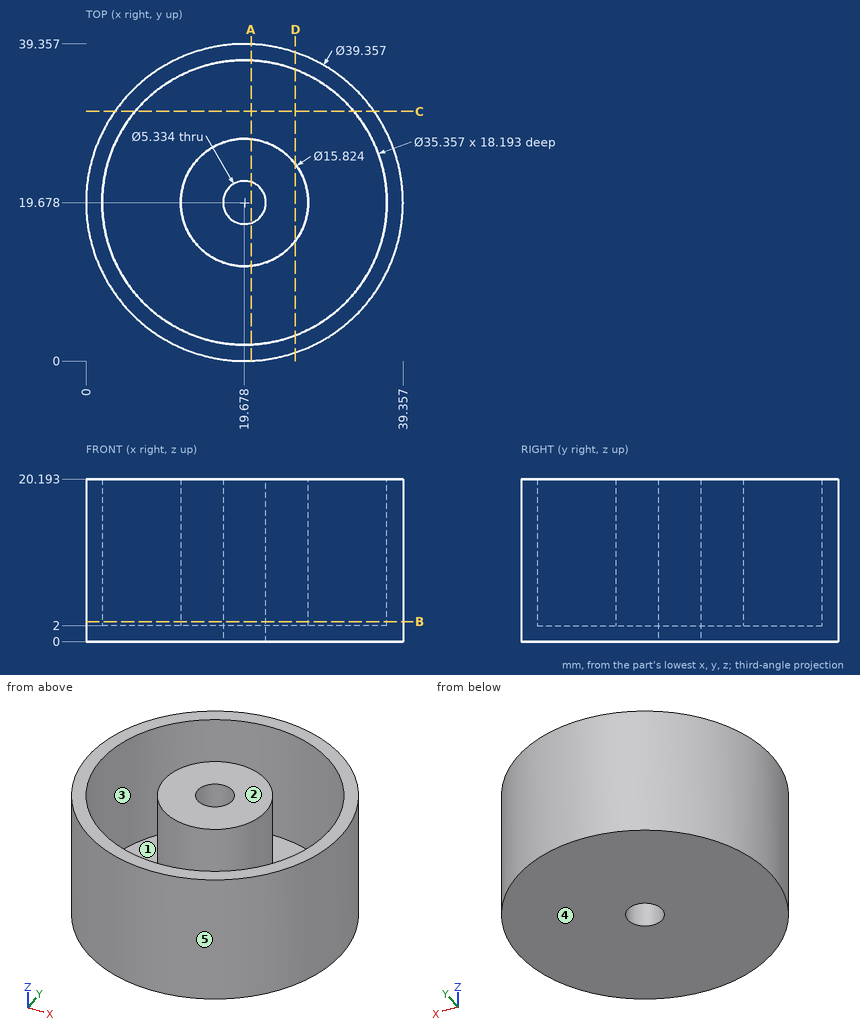
Check sheet for the drawn part. Datum: minimum x, y, z corner. Units: mm. A direction names the side the tool comes from. Give positions to 0.01 mm unless a question says otherwise; leave off trailing zeros. Loops run counter-clockwise (first coordinate to the right, second up) from the corner with the lowest first, then second, coordinate; pieces in that order, holes last. Notation, with made-up numbers: M -4,64.25 L 29,64.25 A24 ccw 29,96.25 Z; hole C 16,-13 d9. An arc over 180 degrees is marked long. Return JSON: item names as keys, results as strings.
1) Section check B-B, the plane z = 2.5. Enter the section's corners in (x, y) (1 decimal).
Findings:
{"outline": "C 19.7,19.7 d39.4; C 19.7,19.7 d15.8; hole C 19.7,19.7 d35.4; hole C 19.7,19.7 d5.3"}
2) Material ranges on L1, parallel to X at y = 26, z = 4.5 (1 decimal); L2, parallel to X at y = 14.5, z = 13.75 (1 decimal); L3, parallel to Y at x = 13.5, z = 17.5 (1 decimal), recorded low to high. Write a range as [from, to].
Findings:
{"L1": "x = [1, 3.2], [14.9, 24.4], [36.2, 38.3]", "L2": "x = [0.7, 2.8], [13.7, 25.7], [36.6, 38.7]", "L3": "y = [1, 3.1], [14.7, 24.6], [36.2, 38.4]"}
3) Section check C-C, the plane y = 31. Enter the section's corners in (x, z).
Findings:
{"outline": "M 3.58,0 L 35.77,0 L 35.77,20.19 L 33.26,20.19 L 33.26,2 L 6.1,2 L 6.1,20.19 L 3.58,20.19 Z"}
4) Gauge pin test, flat ends, axial feed: P1, Ø1, axis at x = 30, y = 10.5, coming from the +Z side; P2, Ø3, axis at x = 25.5, z = 7.5, coming from the +Y side; P3, Ø3, axis at y = 31, z = 5, coming from the +X side; P4, Ø4.5, axis at x = 19.68, y = 19.68, coming from the -Z side. Record the tip position at first contact, or that the pin passes through.
Findings:
{"P1": "stops at z = 2", "P2": "stops at y = 38.88", "P3": "stops at x = 36.73", "P4": "passes through"}
5) Mould release check, pull along X, two halves, no side actions. Record for the marked faces 3, 4 and 5: released by +X, released by -X, zero draft, split by the parting line, or undercut.
Findings:
{"face 3": "undercut", "face 4": "zero draft", "face 5": "split by the parting line"}
6) Section check D-D, the plane x = 26. Enter the section's corners in (y, z), and give its area (3 significant figures).
Findings:
{"outline": "M 1.04,0 L 38.31,0 L 38.31,20.19 L 36.19,20.19 L 36.19,2 L 24.44,2 L 24.44,20.19 L 14.92,20.19 L 14.92,2 L 3.17,2 L 3.17,20.19 L 1.04,20.19 Z", "area": "325 mm2"}
7) Tool access check on the marked faces 1 and 2. Record the directions out of +Z, -Z, +X, -X, +Y, -Y that give a thin tool (end or side, any length) a straight path to the whole face; none if there is none.
Findings:
{"face 1": "+Z", "face 2": "+Z, +X, -X, +Y, -Y"}
8) Section check A-A, the plane x = 20.5. Enter the section's corners in (y, z) (1 decimal).
Findings:
{"outline": "M 0,0 L 17.1,0 L 17.1,20.2 L 11.8,20.2 L 11.8,2 L 2,2 L 2,20.2 L 0,20.2 Z; M 22.2,0 L 39.3,0 L 39.3,20.2 L 37.3,20.2 L 37.3,2 L 27.5,2 L 27.5,20.2 L 22.2,20.2 Z"}
